from build123d import *

# Parameters (mm, degrees)
ESQUISSE1_R      = 5.6
EXTRUSION1_DEPTH = 2.5
ESQUISSE2_R      = 9.5
EXTRUSION2_DEPTH = 1.5
ESQUISSE3_R      = 1.5
EXTRUSION3_DEPTH = 31.141796481


with BuildPart() as part:
    # Esquisse1 → Extrusion1 (new body)
    with BuildSketch(Plane.XY):
        with BuildLine():
            Line((-22, 9.451843318), (-22, -3.548156682))
            Line((-22, -3.548156682), (0, -3.548156682))
            Line((0, -3.548156682), (0, 9.451843318))
            ThreePointArc((0, 9.451843318), (-11, 20.451843318), (-22, 9.451843318))
        make_face()
        with Locations((-11, 9.451843318)):
            Circle(ESQUISSE1_R, mode=Mode.SUBTRACT)
    extrude(amount=EXTRUSION1_DEPTH)

    # Esquisse2 → Extrusion2 (cut)
    with BuildSketch(Plane.XY.offset(2.5)):
        with Locations((-11, 9.451843318)):
            Circle(ESQUISSE2_R)
    extrude(amount=-EXTRUSION2_DEPTH, mode=Mode.SUBTRACT)

    # Esquisse3 → Extrusion3 (cut, through all)
    with BuildSketch(Plane.XY.offset(2.5)):
        with Locations((-19.5, -1.048156682)):
            Circle(ESQUISSE3_R)
    extrude(amount=-EXTRUSION3_DEPTH, mode=Mode.SUBTRACT)


solid = part.part
Could you check a few things on this model? Use its own coordinates, in mm. A direction names the side the tool comes from. Give positions to 0.01 mm unless a question says otherwise; leave off trailing zeros. Order: outer loops, then holes, each group sorted by start corner. A loop starts at its lowest first (then second) coordinate and runs counter-clockwise, first axis right, second up. Notation, with made-up numbers: (10, 89) -> (54, 89) arc R18 cw to (54, 102) -> close; hole circle Ø6 at (-11.75, 79.5). An arc over 180 degrees is marked (long way). Answer in a Markdown table with one row per item. Add a question column.
Item 1: Imagine slicing it at A-A (x = -11). List the corners of the cut face in (y, z) for me.
Item 2: Imagine slicing it at D-D (y = -1.5). List the corners of the cut face in (x, z) for me.
Item 3: Imagine slicing it at C-C (z = 1.8). List the corners of the cut face in (x, y) for me, and give its area (3 significant figures).
Item 4: For faces 1 (the cylindrical face through (-13.059, 0.178, 1.76)), 2 (the flat face through (0, 3, 1)), which set-ups out of +Z, -Z, +X, -X, +Y, -Y let a thin tool reach every point of the face, with its end or its side?
Item 5: Please list where these lines run through material, in increasing order: probe 1 along Y at (x, z) = (-11, 0.35); probe 2 along X at (y, z) = (9.5, 0.2); probe 3 along Z at (x, y) = (-4, 8.5).
Item 6: We'd pull the mould along Y, two halves only. Please class faces 3 (the flat face through (-11, -3.548, 1)), 4 (the flat face through (-7, 5, 1)), 5 (the flat face through (-11, 3, 0)): pulls with the +Y half, pulls with the -Y half, needs draft (parallel to the pull), parting line crosses it, or undercut.
Item 7: I'm going to push flat-ended pins straight in: P1, Ø4, axis at x = -19.5, y = -1.05, coming from the -Z side; P2, Ø9, axis at x = -11, y = 9.45, coming from the -Z side. Where does each tip first touch, or does it pass through?
Item 8: Imagine slicing it at B-B (y = 12). List the corners of the cut face in (x, z) for me.
Result:
| question | item | result |
|---|---|---|
| 1 | outline | (-3.55, 0) -> (3.85, 0) -> (3.85, 1) -> (-0.05, 1) -> (-0.05, 2.5) -> (-3.55, 2.5) -> close; (15.05, 0) -> (20.45, 0) -> (20.45, 2.5) -> (18.95, 2.5) -> (18.95, 1) -> (15.05, 1) -> close |
| 2 | outline | (-22, 0) -> (-20.93, 0) -> (-20.93, 2.5) -> (-22, 2.5) -> close; (-18.07, 0) -> (0, 0) -> (0, 2.5) -> (-18.07, 2.5) -> close |
| 3 | outline | (-22, -3.55) -> (0, -3.55) -> (0, 9.45) arc R11 ccw to (-22, 9.45) -> close; hole circle Ø3 at (-19.5, -1.05); hole circle Ø19 at (-11, 9.45) |
| 3 | area | 185 mm2 |
| 4 | face 1 | +Z |
| 4 | face 2 | +Z, -Z, +X, +Y, -Y |
| 5 | probe 1 | -3.55 to 3.85, 15.05 to 20.45 |
| 5 | probe 2 | -22 to -16.6, -5.4 to 0 |
| 5 | probe 3 | 0 to 1 |
| 6 | face 3 | pulls with the -Y half |
| 6 | face 4 | undercut |
| 6 | face 5 | needs draft |
| 7 | P1 | z = 0 |
| 7 | P2 | through |
| 8 | outline | (-21.7, 0) -> (-15.99, 0) -> (-15.99, 1) -> (-20.15, 1) -> (-20.15, 2.5) -> (-21.7, 2.5) -> close; (-6.01, 0) -> (-0.3, 0) -> (-0.3, 2.5) -> (-1.85, 2.5) -> (-1.85, 1) -> (-6.01, 1) -> close |
